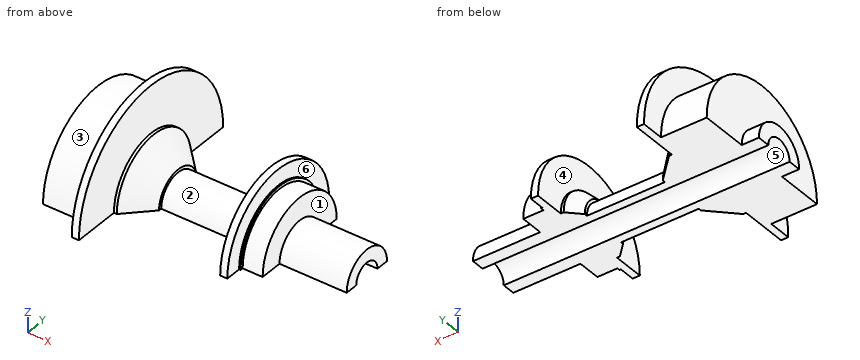
from build123d import *

# Parameters (mm, degrees)
REVOLUTION_ANGLE = 180


with BuildPart() as part:
    # Sketch → Revolution (revolve)
    with BuildSketch(Plane.XY):
        Polygon((26.5, 9.5), (26.5, 17.46), (19.5, 17.46), (19.5, 18.46), (19, 18.46), (19, 24), (16.5, 24), (16.5, 13.242641), (15.5, 13.242641), (11.257359, 9), (11.257359, 8), (-16.014719, 8), (-16.014719, 9), (-24.5, 17.485281), (-25.5, 17.485281), (-25.5, 34), (-28, 34), (-28, 26), (-44, 26), (-44, 9.5), (-50, 9.5), (-50, 5), (50, 5), (50, 9.5), align=None)
    revolve(axis=Axis((0, 0, 0), (1, 0, 0)), revolution_arc=REVOLUTION_ANGLE)


solid = part.part
CAD build for the part. Positions are in the model's coordinates, mm. Face numbers are marked on the shaded views. A direction names the side the tool comes from. Give positions to 0.01 mm unless a question says otherwise; leave off trailing zeros. Loops run counter-clockwise (first coordinate to the right, second up) from the corner with the lowest first, then second, coordinate; pieces in that order, holes last. Notation, with made-up numbers: M 25.25,-23 L 34.25,-23 A25 cw 34.25,8 Z; hole C 43.5,39 d4. An arc over 180 degrees is marked long. One line per question, with ' | ' between items. Start each with the question number.
1. 3-axis set-ups, long thin cutter, end or side, ignore diameter. For the marked faces 1, 2 and 3: which of +Z, -Z, +X, -X, +Y, -Y reach the whole face in a straight line?
2. Two-plate mould, pull along X, no slides. Class the marked faces 4, 5 and 6: pulls with the +X half, pulls with the -X half, needs draft (parallel to the pull), parting line crosses it, or undercut.
3. Saw through at A-A on y = 0. Give the cut face in (x, z).
4. Probe L1, parallel to X at y = 16, z = 20; L2, parallel to X at y = -4.5, z = 9; L3, parallel to X at y = 30.5, z = 1.5. List the from-to ranges inside material, lowest first. Write a range as from..to.
5. Flat gauge pins, fed straight in: pin 1 (8 mm diameter, centred on x = 12, z = 3.5, fed in from -Y); pin 2 (3 mm diameter, centred on y = -17, z = 29.5, fed in from +X); pin 3 (3 mm diameter, centred on y = 18, z = 28, fed in from -X). Where does each tip first touch, or does it go through?
6. Saw through at C-C on z = 31.5. Give the cut face in (x, y), plus the area to 3 significant figures.
7. Saw through at B-B on x = -36.5. Give the cut face in (y, z).
Result sheet:
1) face 1: +Z, +X | face 2: +Z | face 3: +Z, -X
2) face 4: undercut | face 5: needs draft | face 6: pulls with the +X half
3) outline: M -50,5 L 50,5 L 50,9.5 L 26.5,9.5 L 26.5,17.46 L 19.5,17.46 L 19.5,18.46 L 19,18.46 L 19,24 L 16.5,24 L 16.5,13.24 L 15.5,13.24 L 11.26,9 L 11.26,8 L -16.01,8 L -16.01,9 L -24.5,17.49 L -25.5,17.49 L -25.5,34 L -28,34 L -28,26 L -44,26 L -44,9.5 L -50,9.5 Z
4) L1: x = -44..-25.5 | L2: x = -44..-17.08, 12.32..26.5 | L3: x = -28..-25.5
5) pin 1: stops at y = -13.15 | pin 2: stops at x = -25.5 | pin 3: stops at x = -28
6) outline: M -28,-12.8 L -25.5,-12.8 L -25.5,12.8 L -28,12.8 Z | area: 64.0 mm^2
7) outline: M -26,0 L -5,0 A5 cw 5,0 L 26,0 A26 ccw Z
